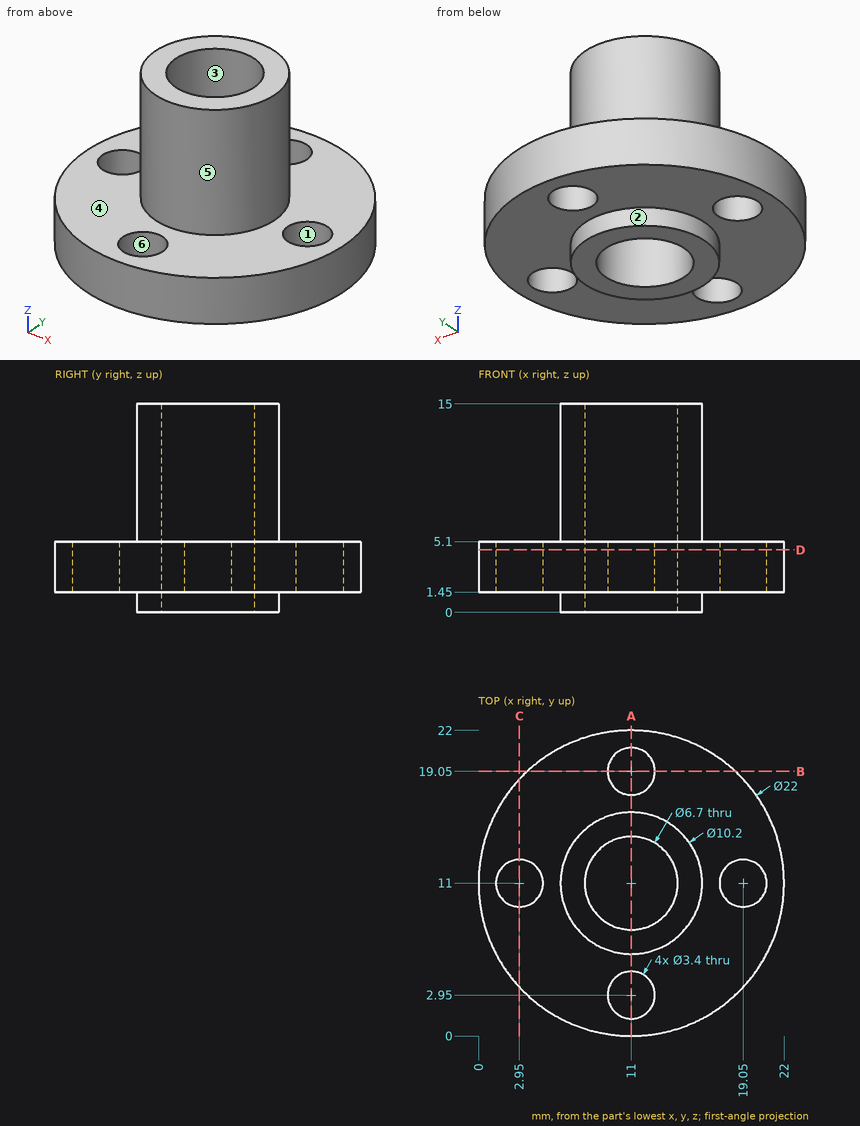
The figure shows three views and two pictorial views of one solid part (mm, origin at its lowest corner). Answer the questions. A direction names the side the tool comes from. Coordinates: 2 decimals unless noted, no trailing zeros. Loops run counter-clockwise (first coordinate to the right, second up) from the corner with the lowest first, then second, coordinate; pieces in that order, holes last. Notation, with made-up numbers: (47, 25.25) - (74, 25.25) arc R14 cw to (74, 29.25) - close; hole circle Ø11 at (-8, 9). An arc over 180 degrees is marked (long way). Write item = value, one per line.
1) Determine the mould class of the marked faces 3, 4, 5 and 6 for opening direction Y: pulls with the +Y half, pulls with the -Y half, needs draft (parallel to the pull), parting line crosses it, or undercut.
Responses:
face_3 = undercut
face_4 = needs draft
face_5 = parting line crosses it
face_6 = undercut
2) Section B-B (y = 19.05) is taken. Determine the outline of the cut face in (x, z), plus the area to 3 significant figures.
Responses:
outline = (3.5, 1.45) - (9.3, 1.45) - (9.3, 5.1) - (3.5, 5.1) - close; (12.7, 1.45) - (18.5, 1.45) - (18.5, 5.1) - (12.7, 5.1) - close
area = 42.3 mm^2
3) Find the intervals of material crossed by line 1 along Y through (x, z) = (11, 3.9); line 2 along Y through (x, z) = (12, 5); line 3 along Z through (x, y) = (17.25, 7), in increasing order.
Responses:
line_1 = 0 to 1.25, 4.65 to 7.65, 14.35 to 17.35, 20.75 to 22
line_2 = 0.05 to 1.58, 4.32 to 7.8, 14.2 to 17.68, 20.42 to 21.95
line_3 = 1.45 to 5.1
4) Section A-A (x = 11) is taken. Determine the outline of the cut face in (y, z).
Responses:
outline = (0, 1.45) - (1.25, 1.45) - (1.25, 5.1) - (0, 5.1) - close; (4.65, 1.45) - (5.9, 1.45) - (5.9, 0) - (7.65, 0) - (7.65, 15) - (5.9, 15) - (5.9, 5.1) - (4.65, 5.1) - close; (14.35, 0) - (16.1, 0) - (16.1, 1.45) - (17.35, 1.45) - (17.35, 5.1) - (16.1, 5.1) - (16.1, 15) - (14.35, 15) - close; (20.75, 1.45) - (22, 1.45) - (22, 5.1) - (20.75, 5.1) - close
5) Each of these flat-tipped pins is pushed along its axis until it touches: P1, Ø3, axis at y = 4.5, z = 5.5, coming from the +X side; P2, Ø1, axis at x = 3.5, y = 3, coming from the +Z side; P3, Ø1.5, axis at y = 15, z = 3, coming from the -X side. Where does it stop, or does it pass through?
Responses:
P1 = 20.77
P2 = 5.1
P3 = 0.49
6) Which of the six approach directions +Z, -Z, +X, -X, +Y, -Y give full straight-line access (tool end or side, diameter ignored) to the marked faces 1 and 2?
Responses:
face_1 = +Z, -Z
face_2 = -Z
7) Section D-D (z = 4.5) is taken. Determine the outline of the cut face in (x, y), plus the area to 3 significant figures.
Responses:
outline = circle Ø22 at (11, 11); hole circle Ø3.4 at (2.95, 11); hole circle Ø6.7 at (11, 11); hole circle Ø3.4 at (11, 2.95); hole circle Ø3.4 at (11, 19.05); hole circle Ø3.4 at (19.05, 11)
area = 309 mm^2
